```python
from build123d import *

# Parameters (mm, degrees)
SKETCH1_R           = 5
BOSS_EXTRUDE2_DEPTH = 13.5
SKETCH3_R           = 22.5
SKETCH3_R_2         = 19.136659322
BOSS_EXTRUDE3_DEPTH = 11
SKETCH4_R           = 20
SKETCH4_R_2         = 4.293447478
BOSS_EXTRUDE4_DEPTH = 2.5


with BuildPart() as part:
    # Sketch1 → Boss-Extrude2 (new body)
    with BuildSketch(Plane.XY.offset(1381.117015566)):
        with Locations((622.689594412, 901.072344281)):
            Circle(SKETCH1_R)
        with BuildLine():
            Line((621.366718756, 902.572344281), (624.012470067, 902.572344281))
            ThreePointArc((624.012470067, 902.572344281), (622.689594412, 899.072344281), (621.366718756, 902.572344281))
        make_face(mode=Mode.SUBTRACT)
    extrude(amount=BOSS_EXTRUDE2_DEPTH)



with BuildPart() as body_2:
    # Sketch3 → Boss-Extrude3 (new, symmetric)
    with BuildSketch(Plane.XY.offset(1392.117015566)):
        with Locations((622.689594412, 901.072344281)):
            Circle(SKETCH3_R)
        with Locations((622.689594412, 901.072344281)):
            Circle(SKETCH3_R_2, mode=Mode.SUBTRACT)
    extrude(amount=BOSS_EXTRUDE3_DEPTH, both=True)


with BuildPart() as part_1:
    add(part.part)

    add(body_2.part)  # Boss-Extrude4 merges body 2
    # Sketch4 → Boss-Extrude4 (add, symmetric)
    with BuildSketch(Plane.XY.offset(1392.117015566)):
        with Locations((622.689594412, 901.072344281)):
            Circle(SKETCH4_R)
        with Locations((622.689594412, 901.072344281)):
            Circle(SKETCH4_R_2, mode=Mode.SUBTRACT)
    extrude(amount=BOSS_EXTRUDE4_DEPTH, both=True)


solid = part_1.part
```
Can you work these out from the model? Positions are in its coordinate system, mm. A direction names the side the tool comes from. Round coordinates to 2 decimals unless told otherwise and drop trailing zeros. Order: outer loops, then holes, each group sorted by start corner. A loop starts at its lowest first (then second) coordinate and runs counter-clockwise, first axis right, second up. Notation, with made-up numbers: (4, 38) -> (58, 38) arc R28 cw to (58, 60) -> close; hole circle Ø6 at (68, 41.5). An arc over 180 degrees is marked (long way). Return JSON: item names as keys, results as strings. Group by question number.
1. If we section it at B-B, the plane y = 890.5: Write out the boundary of the cut face in (x, z), then the cut area to 3 significant figures.
2. If we section it at A-A, the plane z = 1388.5: Write out the boundary of the cut face in (x, y).
3. Will these pins go through, and if not, where does the flat tip stop? pin 1 (1.3 mm diameter, centred on x = 623, z = 1386, fed in from -Y); pin 2 (11.5 mm diameter, centred on x = 613.5, y = 891.5, fed in from -Z); pin 3 (2 mm diameter, centred on y = 896.5, z = 1391, fed in from -X) (3 decimals).
4. I need wall thicknesses on line 1 (Y direction, x = 622.5, z = 1382.25); line 2 (X direction, y = 900.5, z = 1397.75); line 3 (Z direction, x = 615.5, y = 887). Which ranges of each line are inside material? Lowest first, please. Write a range as [from, to].
5. We'd pull the mould along X, two halves only. Please class faces 4 (the face through (629, 920, 1381.117)), 5 (the face through (617.812, 879.107, 1392.271)), 6 (the face through (623, 902.572, 1388)): released by +X, released by -X, zero draft, split by the parting line, or undercut.
6. If we section it at C-C, the plane x = 612: Write out the boundary of the cut face in (y, z), then the cut area to 3 significant figures.
7. If we section it at D-D, the plane z = 1391: Write out the boundary of the cut face in (x, y), then the cut area to 3 significant figures.
8. Which directions (+Z, -Z, +X, -X, +Y, -Y) give clear straight access to the entire face, cutting with the end or side of a thin tool? Please do faces 1 (the face through (629, 920, 1403.117)), 2 (the face through (618.5, 882.4, 1385.3)), 3 (the face through (618.5, 882.4, 1398.8)).
Output values:
{
 "1": {"outline": "(602.83, 1381.12) -> (606.74, 1381.12) -> (606.74, 1389.62) -> (638.64, 1389.62) -> (638.64, 1381.12) -> (642.55, 1381.12) -> (642.55, 1403.12) -> (638.64, 1403.12) -> (638.64, 1394.62) -> (606.74, 1394.62) -> (606.74, 1403.12) -> (602.83, 1403.12) -> close", "area": "332 mm²"},
 "2": {"outline": "circle Ø45 at (622.69, 901.07); circle Ø10 at (622.69, 901.07); hole circle Ø38.27 at (622.69, 901.07); hole (621.37, 902.57) arc R2 ccw (long way) to (624.01, 902.57) -> close"},
 "3": {"pin 1": "y = 878.57", "pin 2": "z = 1389.62", "pin 3": "x = 600.475"},
 "4": {"line 1": "[878.57, 881.94], [896.08, 899.08], [902.57, 906.07], [920.21, 923.57]", "line 2": "[600.2, 603.56], [641.82, 645.18]", "line 3": "[1389.62, 1394.62]"},
 "5": {"face 4": "zero draft", "face 5": "split by the parting line", "face 6": "undercut"},
 "6": {"outline": "(881.27, 1381.12) -> (885.2, 1381.12) -> (885.2, 1389.62) -> (916.95, 1389.62) -> (916.95, 1381.12) -> (920.87, 1381.12) -> (920.87, 1403.12) -> (916.95, 1403.12) -> (916.95, 1394.62) -> (885.2, 1394.62) -> (885.2, 1403.12) -> (881.27, 1403.12) -> close", "area": "331 mm²"},
 "7": {"outline": "circle Ø45 at (622.69, 901.07); hole (621.37, 902.57) arc R2 ccw (long way) to (624.01, 902.57) -> close", "area": "1,580 mm²"},
 "8": {"face 1": "+Z, +X, -X, +Y, -Y", "face 2": "-Z", "face 3": "+Z"}
}
